```python
from build123d import *

# Parameters (mm, degrees)
SKETCH1_R               = 12.5
BOSS_EXTRUDE2_DEPTH     = 38.5
SKETCH3_R               = 14
BOSS_EXTRUDE3_DEPTH     = 5
CUT_EXTRUDE1_DEPTH      = 44.292609069
CUT_EXTRUDE1_DEPTH_BACK = 7
SKETCH4_R               = 11.05
SKETCH5_R               = 7.5
CUT_EXTRUDE2_DEPTH      = 7
FILLET2_R               = 3
FILLET3_R               = 1.5
CHAMFER1_SIZE           = 1


with BuildPart() as part:
    # Sketch1 → Boss-Extrude2 (new body)
    with BuildSketch(Plane(origin=(0, 0, 0), x_dir=(0, 0, -1), z_dir=(1, 0, 0))):
        Circle(SKETCH1_R)
    extrude(amount=BOSS_EXTRUDE2_DEPTH)

    # Sketch3 → Boss-Extrude3 (add)
    with BuildSketch(Plane(origin=(38.5, 0, 0), x_dir=(0, 0, -1), z_dir=(1, 0, 0))):
        Circle(SKETCH3_R)
    extrude(amount=-BOSS_EXTRUDE3_DEPTH)

    # Sketch4 → Cut-Extrude1 (cut, two sides: drawn at the far end of the back side and taken through both)
    with BuildSketch(Plane(origin=(38.5, 0, 0), x_dir=(0, 0, -1), z_dir=(1, 0, 0)).offset(-CUT_EXTRUDE1_DEPTH_BACK)):
        with Locations(Location((0, 0, 0), (0, 0, 180))):
            Circle(SKETCH4_R)
    extrude(amount=CUT_EXTRUDE1_DEPTH + CUT_EXTRUDE1_DEPTH_BACK, mode=Mode.SUBTRACT)

    # Sketch5 → Cut-Extrude2 (cut)
    with BuildSketch(Plane(origin=(31.5, 0, 0), x_dir=(0, 0, -1), z_dir=(1, 0, 0))):
        Circle(SKETCH5_R)
    extrude(amount=-CUT_EXTRUDE2_DEPTH, mode=Mode.SUBTRACT)

    # Fillet2
    # the kernel refuses this fillet: 3 mm, written as the material it adds along each edge
    with BuildSketch(Plane(origin=(33.5, 0, 0), x_dir=(0, 0, -1), z_dir=(0, 1, 0))) as fillet2_piece_1:
        with BuildLine():
            CenterArc((15.5, 2.598076211), FILLET2_R, 180, 60)
            Line((14, 0), (13.97, -0.051961524))
            ThreePointArc((13.97, -0.051961524), (13.25, -0.06), (12.5, -0.06))
            Line((12.5, -0.06), (12.44, 0))
            Line((12.44, 0), (12.44, 2.598076211))
            Line((12.44, 2.598076211), (12.5, 2.598076211))
        make_face()
    revolve(axis=Axis((33.5, 0, 0), (-1, 0, 0)))

    # Fillet3
    fillet3_edges = [part.edges().sort_by_distance(p)[0] for p in [
        (33.5, 0, 14),
        (38.5, 0, 14),
    ]]
    fillet(fillet3_edges, radius=FILLET3_R)

    # Mirror1: part across plane


with BuildPart() as part_1:
    add(part.part)
    add(part.part.mirror(Plane(origin=(0, 0, 0), x_dir=(0, 0, 1), z_dir=(1, 0, 0))))

    # Chamfer1
    chamfer1_edges = [part_1.edges().sort_by_distance(p)[0] for p in [
        (24.5, 0, 7.5),
        (31.5, 0, 7.5),
    ]]
    chamfer(chamfer1_edges, length=CHAMFER1_SIZE)


solid = part_1.part
```
Verification items for the finished model (mm, model axes). A direction names the side the tool comes from. Give positions to 0.01 mm unless a question says otherwise; leave off trailing zeros. Loops run counter-clockwise (first coordinate to the right, second up) from the corner with the lowest first, then second, coordinate; pieces in that order, holes last. Notation, with made-up numbers: M 32,28 L 76,28 A18 cw 76,38 Z; hole C 17.5,-37.5 d7. An arc over 180 degrees is marked long. Return JSON: item names as keys, results as strings.
1) Section check A-A, the plane x = -14.5. Enter the section's corners in (y, z).
Findings:
{"outline": "C 0,0 d25"}
2) Mould release check, pull along Y, two halves, no side actions. Record for faces 5 (the conical face through (31, 0, 8)), 6 (the cylindrical face through (-35.65, 4.21, -13.35)), 7 (the flat face through (38.5, -9.2, -6.4)): released by +Y, released by -Y, zero draft, split by the parting line, or undercut.
Findings:
{"face 5": "undercut", "face 6": "split by the parting line", "face 7": "zero draft"}
3) Tool access check on faces 1 (the cylindrical face through (-0.433, 3.755, -11.923)), 2 (the flat face through (-24.5, 0, 0)), 3 (the cylindrical face through (34.95, 6.72, -8.77)), 4 (the flat face through (-38.5, -9.2, -6.4)). Record the directions out of +Z, -Z, +X, -X, +Y, -Y that give a thin tool (end or side, any length) a straight path to the whole face; none if there is none.
Findings:
{"face 1": "none", "face 2": "-X", "face 3": "+X", "face 4": "+Z, -Z, -X, +Y, -Y"}
4) Gauge pin test, flat ends, axial feed: P1, Ø3, axis at x = 10, y = 3, coming from the -Z side; P2, Ø10, axis at x = -4, y = 1, coming from the -Z side; P3, Ø3, axis at x = 13, z = 0, coming from the +Y side. Record the tip position at first contact, or that the pin passes through.
Findings:
{"P1": "stops at z = -12.41", "P2": "stops at z = -12.5", "P3": "stops at y = 12.5"}
5) Material ranges on L1, parallel to Y at x = 27.6, z = 0; L2, parallel to X at y = 3.75, z = 3.25; L3, parallel to X at y = 7.25, z = -7.5, recorded low to high. Write a range as [from, to].
Findings:
{"L1": "y = [-12.5, -7.5], [7.5, 12.5]", "L2": "x = [-24.5, 24.5]", "L3": "x = [-31.5, 31.5]"}
